```python
from build123d import *

# Parameters (mm, degrees)
SKETCH1_W           = 150
SKETCH1_H           = 30
BOSS_EXTRUDE1_DEPTH = 10
SKETCH9_W           = 150
SKETCH9_H           = 250
SKETCH9_W_2         = 100
SKETCH9_H_2         = 100
BOSS_EXTRUDE3_DEPTH = 10
SKETCH25_W          = 150
SKETCH25_H          = 30
CUT_EXTRUDE2_DEPTH  = 10


with BuildPart() as part:
    # Sketch1 → Boss-Extrude1 (new body)
    with BuildSketch(Plane(origin=(0, 0, 0), x_dir=(1, 0, 0), z_dir=(0, 1, 0))):
        with Locations((-75, 15)):
            Rectangle(SKETCH1_W, SKETCH1_H)
    extrude(amount=BOSS_EXTRUDE1_DEPTH)

    # Sketch9 → Boss-Extrude3 (add)
    with BuildSketch(Plane.XZ):
        with Locations((-75, -15)):
            Rectangle(SKETCH9_W, SKETCH9_H)
        with Locations((-75, -15)):
            Rectangle(SKETCH9_W_2, SKETCH9_H_2, mode=Mode.SUBTRACT)
    extrude(amount=BOSS_EXTRUDE3_DEPTH)

    # Sketch25 → Cut-Extrude2 (cut)
    with BuildSketch(Plane(origin=(0, 0, 0), x_dir=(1, 0, 0), z_dir=(0, 1, 0))):
        with Locations((-75, 15)):
            Rectangle(SKETCH25_W, SKETCH25_H)
    extrude(amount=CUT_EXTRUDE2_DEPTH, mode=Mode.SUBTRACT)


solid = part.part
```
Check sheet for the modelled part. Datum: model origin and axes. Units: mm. A direction names the side the tool comes from. Give positions to 0.01 mm unless a question says otherwise; leave off trailing zeros. Order: outer loops, then holes, each group sorted by start corner. A loop starts at its lowest first (then second) coordinate and runs counter-clockwise, first axis right, second up. Notation, with made-up numbers: (88, -38) -> (139, -38) arc R18 cw to (139, -3) -> close; hole circle Ø2 at (-35, 14). An arc over 180 degrees is marked (long way). Return JSON: item names as keys, results as strings.
1. Material ranges on probe 1 along Z at (x, y) = (-64, -1); probe 2 along X at (y, z) = (-3, 31), recorded low to high. Write a range as [from, to].
From the geometry:
{"probe 1": "[-140, -65], [35, 110]", "probe 2": "[-150, -125], [-25, 0]"}
2. Cross-section at B-B, the plane x = -68.5. Record the cut outline in (y, z), plus the area to 3 significant figures.
From the geometry:
{"outline": "(-10, -140) -> (0, -140) -> (0, -65) -> (-10, -65) -> close; (-10, 35) -> (0, 35) -> (0, 110) -> (-10, 110) -> close", "area": "1,500 mm^2"}
3. Mould release check, pull along Z, two halves, no side actions. Record for faces 1 (the flat face through (-25, -5, -16)), 2 (the flat face through (-150, -5, -17)), 3 (the flat face through (-76, -5, 110)): +Z half, -Z half, draft (parallel to the pull), parting line (faces both ways), or undercut.
From the geometry:
{"face 1": "undercut", "face 2": "draft", "face 3": "+Z half"}
4. Set-up check for faces 4 (the flat face through (-76, -5, -140)), 5 (the flat face through (-125, -5, -16)): record each of +Z, -Z, +X, -X, +Y, -Y from which the full face is reachable in a straight line by a thin tool's end or side.
From the geometry:
{"face 4": "-Z, +X, -X, +Y, -Y", "face 5": "+Y, -Y"}
5. Cross-section at A-A, the plane y = -8. Record the cut outline in (x, z).
From the geometry:
{"outline": "(-150, -140) -> (0, -140) -> (0, 110) -> (-150, 110) -> close; hole (-125, -65) -> (-25, -65) -> (-25, 35) -> (-125, 35) -> close"}
6. Cross-section at C-C, the plane z = -38. Record the cut outline in (x, y).
From the geometry:
{"outline": "(-150, -10) -> (-125, -10) -> (-125, 0) -> (-150, 0) -> close; (-25, -10) -> (0, -10) -> (0, 0) -> (-25, 0) -> close"}
